from build123d import *

# Parameters (mm, degrees)
BOSS_EXTRUDE1_DEPTH = 15
SKETCH5_R           = 3
CUT_EXTRUDE1_DEPTH  = 71.242437315


with BuildPart() as part:
    # Sketch2 → Boss-Extrude1 (new, symmetric)
    with BuildSketch(Plane.XY):
        Polygon((-65, 11), (-65, -11), (-39.13, -11), (-37.28, -9.565), (37.28, -9.565), (39.13, -11), (65, -11), (65, 11), (39.13, 11), (37.28, 9.565), (-37.28, 9.565), (-39.13, 11), align=None)
        with BuildLine():
            Line((0, 2.815), (18.655, 2.815))
            ThreePointArc((18.655, 2.815), (31.83, 0), (18.655, -2.815))
            Line((18.655, -2.815), (0, -2.815))
            Line((0, -2.815), (-18.655, -2.815))
            ThreePointArc((-18.655, -2.815), (-31.83, 0), (-18.655, 2.815))
            Line((-18.655, 2.815), (0, 2.815))
        make_face(mode=Mode.SUBTRACT)
    extrude(amount=BOSS_EXTRUDE1_DEPTH, both=True)

    # Sketch5 → Cut-Extrude1 (cut, through all)
    with BuildSketch(Plane(origin=(0, 11, 0), x_dir=(1, 0, 0), z_dir=(0, 1, 0))):
        with Locations(Location((-53, 7.5, 0), (0, 0, 270))):
            Circle(SKETCH5_R)
        with Locations(Location((-53, -7.5, 0), (0, 0, 90))):
            Circle(SKETCH5_R)
        with Locations(Location((53, -7.5, 0), (0, 0, 270))):
            Circle(SKETCH5_R)
        with Locations(Location((53, 7.5, 0), (0, 0, 90))):
            Circle(SKETCH5_R)
    extrude(amount=-CUT_EXTRUDE1_DEPTH, mode=Mode.SUBTRACT)


solid = part.part
Input: part model. Units: mm. Frame: model coordinates. A direction names the side the tool comes from. Round coordinates to 2 decimals unless told otherwise and drop trailing zeros. Order: outer loops, then holes, each group sorted by start corner. A loop starts at its lowest first (then second) coordinate and runs counter-clockwise, first axis right, second up. Notation, with made-up numbers: (6.25, 40) - (40.25, 40) arc R19 cw to (40.25, 58) - close; hole circle Ø2 at (-24, -38). An arc over 180 degrees is marked (long way). Answer as a JSON object with one key per item and string values. Group by question number.
(1) Cut plane B-B (y = 0). Return loops of the section in (x, z).
(2) Cut plane D-D (z = 2). Return loops of the section in (x, y) (3 decimals).
(3) Material intervals for probe 1 along Y at (x, z) = (0, -12) (3 decimals); probe 2 along Y at (x, z) = (-25, -8.5) (3 decimals); probe 3 along X at (y, z) = (-4.75, -12.25), sorted ascending. Write a range as from..to.
(4) Cut plane C-C (x = 53). Return loops of the section in (y, z), then the cut area to 3 significant figures.
(5) Pin query (flat end, axial travel): P1, Ø4, axis at x = -9, z = 5, coming from the +Y side (3 decimals); P2, Ø12, axis at x = -11, z = 5, coming from the -Y side (3 decimals). Return the tip coordinate at first contact, or that it passes through.
(6) Cut plane A-A (z = 7.5). Return loops of the section in (x, y) (3 decimals).
(7) Reachability of faces 1 (the face through (0, -2.815, 0)), 2 (the face through (52, 11, 0)) from +Z, -Z, +X, -X, +Y, -Y: full face, straight path, thin tool, end or side. Return the list, or none.
(8) Draft query along Y for faces 3 (the face through (-31.825, -0.262, 0.21)), 4 (the face through (1, 9.565, 0)), 5 (the face through (50.47, 0.15, -9.11)), 6 (the face through (-1, -9.565, 0)). Return one class per face: released by +Y, released by -Y, zero draft, split by the parting line, or undercut.
Here are the results:
{
 "1": {"outline": "(-65, -15) - (-31.83, -15) - (-31.83, 15) - (-65, 15) - close; (31.83, -15) - (65, -15) - (65, 15) - (31.83, 15) - close; hole circle Ø6 at (-53, -7.5); hole circle Ø6 at (-53, 7.5); hole circle Ø6 at (53, -7.5); hole circle Ø6 at (53, 7.5)"},
 "2": {"outline": "(-65, -11) - (-39.13, -11) - (-37.28, -9.565) - (37.28, -9.565) - (39.13, -11) - (65, -11) - (65, 11) - (39.13, 11) - (37.28, 9.565) - (-37.28, 9.565) - (-39.13, 11) - (-65, 11) - close; hole (-18.655, -2.815) - (18.655, -2.815) arc R6.888 ccw (long way) to (18.655, 2.815) - (-18.655, 2.815) arc R6.888 ccw (long way) to start"},
 "3": {"probe 1": "y = -9.565..-2.815, 2.815..9.565", "probe 2": "y = -9.565..-6.888, 6.888..9.565", "probe 3": "x = -65..-29.93, -19.95..19.95, 29.93..65"},
 "4": {"outline": "(-11, -15) - (11, -15) - (11, -10.5) - (-11, -10.5) - close; (-11, -4.5) - (11, -4.5) - (11, 4.5) - (-11, 4.5) - close; (-11, 10.5) - (11, 10.5) - (11, 15) - (-11, 15) - close", "area": "396 mm^2"},
 "5": {"P1": "stops at y = 9.565", "P2": "stops at y = -9.565"},
 "6": {"outline": "(-65, -11) - (-56, -11) - (-56, 11) - (-65, 11) - close; (-50, -11) - (-39.13, -11) - (-37.28, -9.565) - (37.28, -9.565) - (39.13, -11) - (50, -11) - (50, 11) - (39.13, 11) - (37.28, 9.565) - (-37.28, 9.565) - (-39.13, 11) - (-50, 11) - close; (56, -11) - (65, -11) - (65, 11) - (56, 11) - close; hole (-18.655, -2.815) - (18.655, -2.815) arc R6.888 ccw (long way) to (18.655, 2.815) - (-18.655, 2.815) arc R6.888 ccw (long way) to start"},
 "7": {"face 1": "+Z, -Z", "face 2": "+Z, -Z, +X, -X, +Y"},
 "8": {"face 3": "undercut", "face 4": "released by +Y", "face 5": "zero draft", "face 6": "released by -Y"}
}
